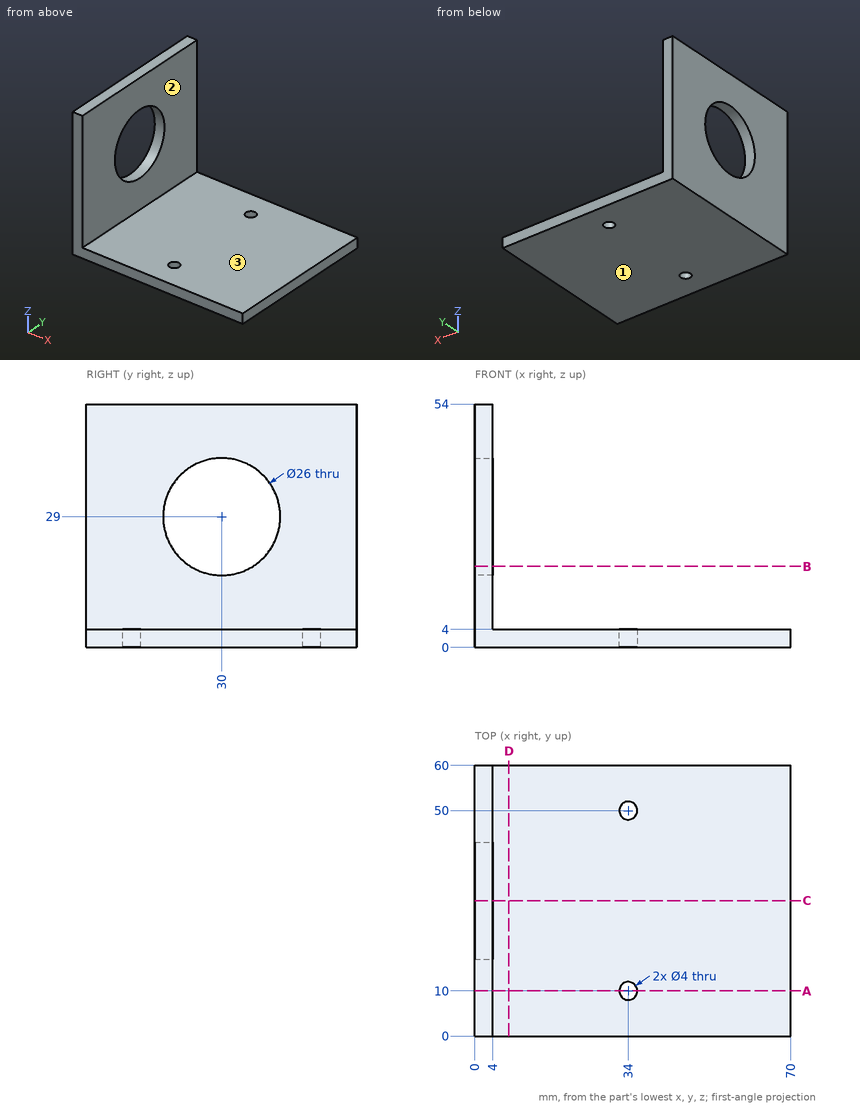
Can you work these out from the drawing? Everything is in mm from the part's minimum corner. Round coordinates to 2 decimals unless told otherwise and drop trailing zeros. Order: outer loops, then holes, each group sorted by start corner. A loop starts at its lowest first (then second) coordinate and runs counter-clockwise, first axis right, second up. Notation, with made-up numbers: (39, 37) - (71, 37) arc R26 cw to (71, 52) - close; hole circle Ø9 at (48, 46). An arc over 180 degrees is marked (long way). Answer in a Markdown table with one row per item.
(1) Suppose I cut it at D-D, the plane x = 7.5. Please give me the cut outline in (y, z).
From the geometry:
| item | result |
|---|---|
| outline | (0, 0) - (60, 0) - (60, 4) - (0, 4) - close |
(2) Suppose I cut it at A-A, the plane y = 10. Please give me the cut outline in (x, z).
From the geometry:
| item | result |
|---|---|
| outline | (0, 0) - (32, 0) - (32, 4) - (4, 4) - (4, 54) - (0, 54) - close; (36, 0) - (70, 0) - (70, 4) - (36, 4) - close |
(3) Suppose I cut it at C-C, the plane y = 30. Please give me the cut outline in (x, z), plus the area to 3 significant figures.
From the geometry:
| item | result |
|---|---|
| outline | (0, 0) - (70, 0) - (70, 4) - (4, 4) - (4, 16) - (0, 16) - close; (0, 42) - (4, 42) - (4, 54) - (0, 54) - close |
| area | 376 mm2 |
(4) For P1, Ø2.5, axis at x = 34, y = 50, coming from the -Z side; P2, Ø6.5, axis at x = 34, y = 10, coming from the +Z side; P3, Ø15, axis at y = 27, z = 38.5, coming from the +X side, each with a flat end and sliding along its axis, tell me the tip position at first contact or that it passes through.
From the geometry:
| item | result |
|---|---|
| P1 | passes through |
| P2 | stops at z = 4 |
| P3 | stops at x = 4 |
(5) Suppose I cut it at B-B, the plane z = 18. Please give me the cut outline in (x, y).
From the geometry:
| item | result |
|---|---|
| outline | (0, 0) - (4, 0) - (4, 23.07) - (0, 23.07) - close; (0, 36.93) - (4, 36.93) - (4, 60) - (0, 60) - close |
(6) Please list where these lines run through material, in increasing order: L1, parallel to Y at x = 34, z = 1.5; L2, parallel to Y at x = 1, z = 29; L3, parallel to X at y = 9.5, z = 8. Write a range as from..to.
From the geometry:
| item | result |
|---|---|
| L1 | y = 0..8, 12..48, 52..60 |
| L2 | y = 0..17, 43..60 |
| L3 | x = 0..4 |
(7) If we mould it in two halves opening along Z, with no side actions, what happens to the marked faces 1, 2 and 3? For each: released by +Z, released by -Z, zero draft, split by the parting line, or undercut.
From the geometry:
| item | result |
|---|---|
| face 1 | released by -Z |
| face 2 | zero draft |
| face 3 | released by +Z |
